Geometry: see drawing. Coordinates: mm, zero at the bounding-box minimum. A direction names the side the tool comes from. Give positions to 0.01 mm unless a question says otherwise; leave off trailing zeros. Loops run counter-clockwise (first coordinate to the right, second up) from the corner with the lowest first, then second, coordinate; pieces in that order, holes last. Notation, with made-up numbers: (41, 65) -> (63, 65) arc R21 ccw to (63, 96) -> close; hole circle Ø7 at (87.25, 66). An arc over 180 degrees is marked (long way). Return JSON: item names as keys, results as strings. Group by question number.
(1) Access query for the marked faces 1 and 2. Directions: +Z, -Z, +X, -X, +Y, -Y. A direction counts if a zero-diameter tool reaches every point of the face in a straight line with its end or side. Return the directions, or none.
(2) Cut plane A-A on y = 29. Return loops of the section in (x, z) (1 decimal).
(3) Cut plane C-C on z = 19.75. Return loops of the section in (x, y).
(4) Cut plane D-D on x = 5.5. Return loops of the section in (y, z) (1 decimal).
(5) Pin query (flat end, axial travel): pin 1 (8 mm diameter, centred on x = 22.5, z = 7.5, fed in from +Y); pin 2 (1 mm diameter, centred on y = 51, z = 1.5, fed in from -X); pin 3 (1 mm diameter, centred on x = 28.5, y = 40, fed in from +Z) (3 decimals). Return the tip coordinate at first contact, or that it passes through.
(6) Ray query, line 1 (Z direction, x = 9, y = 11.5) (1 decimal); line 2 (X direction, y = 42.5, z = 1.25); line 3 (Y direction, x = 7, z = 1.75). Return the intervals inside material, ascending. Write a range as from..to.
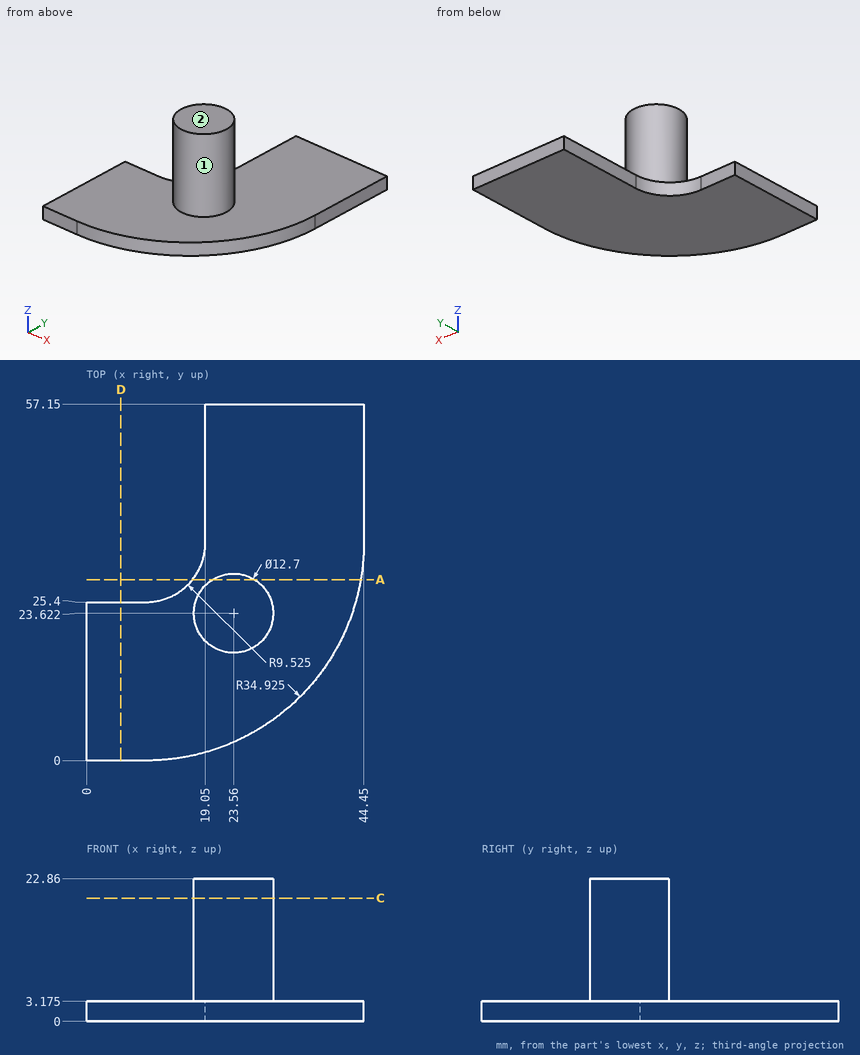
Answers:
{
 "1": {"face 1": "+Z", "face 2": "+Z, +X, -X, +Y, -Y"},
 "2": {"outline": "(17, 0) -> (43.9, 0) -> (43.9, 3.2) -> (26.9, 3.2) -> (26.9, 22.9) -> (20.2, 22.9) -> (20.2, 3.2) -> (17, 3.2) -> close"},
 "3": {"outline": "circle Ø12.7 at (23.56, 23.62)"},
 "4": {"outline": "(0, 0) -> (25.4, 0) -> (25.4, 3.2) -> (0, 3.2) -> close"},
 "5": {"pin 1": "y = 29.97", "pin 2": "x = 19.05", "pin 3": "z = 3.175"},
 "6": {"line 1": "0..3.2", "line 2": "19.05..44.45", "line 3": "0..25.4"}
}
